Geometry: final body of the model. Coordinates: model frame, mm. Give positions to 0.01 mm unless a question says otherwise; leave off trailing zeros. Write each loop counter-clockwise with the first axis right and the second up, starting at its lowest first coordinate (ties: lowest second). Pieces come first, ordered by that corner, then holes. Notation, with made-up numbers: (14.5, 50.25) -> (60.5, 50.25) arc R27 ccw to (60.5, 69.25) -> close; hole circle Ø2 at (86, 23.5). An arc over 180 degrees is marked (long way). Answer as a JSON object with one key per item and string values. Group by question number.
(1) Contact query for flat-ended pins moving along their axis: pin 1 Ø3 at (x, z) = (40, -40) entering from -Y; pin 2 Ø6.5 at (x, z) = (-40, 40) entering from +Y; pin 3 Ø4.5 at (x, z) = (-100.5, -15.5) entering from -Y; pin 4 Ø1 at (x, y) = (188, 3.5) entering from +Z. Output: stop coordinate, or through.
(2) Draft query along X for faces 1 (the face through (61, 5, -1)), 2 (the face through (-104.846, 2.535, -1.465)), 3 (the face through (279, 2, -34)). Return one class per face: +X half, -X half, draft (parallel to the pull), parting line (faces both ways), or undercut.
(3) Section query A-A on y = 3.9. State how many separate pieces and enclosed holes the cut face has, plus the area to 3 significant figures.
(4) Section query B-B on x = 216. Output: boundary loops of the cut face in (y, z).
(5) Material intervals for probe 1 along Z at (x, y) = (-100.5, 2.5); probe 2 along X at (y, z) = (2.8, 15.5); probe 3 along X at (y, z) = (2.2, -1.5), sorted ascending.
(6) Section query C-C on x = 67. Output: boundary loops of the cut face in (y, z), plus the area to 3 significant figures.
from build123d import *

# Parameters (mm, degrees)
BOSS_EXTRUDE2_DEPTH                                 = 5
CHAMFER2_SIZE                                       = 12
FILLET1_R                                           = 7.5
SKETCH2_R                                           = 2.575
SKETCH2_R_2                                         = 11.25
SKETCH2_R_3                                         = 3
CUT_EXTRUDE1_DEPTH                                  = 290.39592257
CSK_FOR_M3_COUNTERSUNK_FLAT_HEAD_SCREW2_D           = 3.4
CSK_FOR_M3_COUNTERSUNK_FLAT_HEAD_SCREW2_CSINK_D     = 6.3
CSK_FOR_M3_COUNTERSUNK_FLAT_HEAD_SCREW2_CSINK_ANGLE = 90


with BuildPart() as part:
    # Sketch1 → Boss-Extrude2 (new body)
    with BuildSketch(Plane(origin=(0, 0, 0), x_dir=(1, 0, 0), z_dir=(0, 1, 0))):
        Polygon((40, -50), (77.320508076, -40), (285, -40), (285, 40), (77.320508076, 40), (40, 50), (-40, 50), (-157, 50), (-157, -50), (-40, -50), align=None)
    extrude(amount=BOSS_EXTRUDE2_DEPTH)

    # Chamfer2
    chamfer2_edges = [part.edges().sort_by_distance(p)[0] for p in [
        (-157, 2.5, 50),
        (-157, 2.5, -50),
        (285, 2.5, -40),
        (285, 2.5, 40),
    ]]
    chamfer(chamfer2_edges, length=CHAMFER2_SIZE)

    # Fillet1
    fillet1_edges = [part.edges().sort_by_distance(p)[0] for p in [
        (40, 2.5, -50),
        (77.320508076, 2.5, -40),
        (77.320508076, 2.5, 40),
        (40, 2.5, 50),
        (-145, 2.5, 50),
        (-157, 2.5, -38),
        (-157, 2.5, 38),
        (-145, 2.5, -50),
        (273, 2.5, -40),
        (285, 2.5, 28),
        (285, 2.5, -28),
        (273, 2.5, 40),
    ]]
    fillet(fillet1_edges, radius=FILLET1_R)

    # Sketch2 → Cut-Extrude1 (cut, through all)
    with BuildSketch(Plane(origin=(0, 5, 0), x_dir=(1, 0, 0), z_dir=(0, 1, 0))):
        with Locations(Location((-40, 40, 0), (0, 0, 270))):
            Circle(SKETCH2_R)
        with Locations(Location((40, 40, 0), (0, 0, 90))):
            Circle(SKETCH2_R)
        with Locations(Location((40, -40, 0), (0, 0, 270))):
            Circle(SKETCH2_R)
        with Locations(Location((-40, -40, 0), (0, 0, 90))):
            Circle(SKETCH2_R)
        with Locations(Location((-116, 0, 0), (0, 0, 270))):
            Circle(SKETCH2_R_2)
        with Locations(Location((0, 0, 0), (0, 0, 270))):
            Circle(SKETCH2_R_3)
    extrude(amount=-CUT_EXTRUDE1_DEPTH, mode=Mode.SUBTRACT)

    # CSK for M3 Countersunk Flat Head Screw2 (through all)
    with Locations(Plane(origin=(0, 0, 0), x_dir=(-1, 0, 0), z_dir=(0, -1, 0))):
        with Locations((131.5, 15.5), (131.5, -15.5), (100.5, -15.5), (100.5, 15.5)):
            CounterSinkHole(CSK_FOR_M3_COUNTERSUNK_FLAT_HEAD_SCREW2_D / 2, CSK_FOR_M3_COUNTERSUNK_FLAT_HEAD_SCREW2_CSINK_D / 2, counter_sink_angle=CSK_FOR_M3_COUNTERSUNK_FLAT_HEAD_SCREW2_CSINK_ANGLE)


solid = part.part
Answer list:
{
 "1": {"pin 1": "through", "pin 2": "y = 5", "pin 3": "y = 0.9", "pin 4": "z = 40"},
 "2": {"face 1": "draft", "face 2": "undercut", "face 3": "+X half"},
 "3": {"separate pieces": "1", "enclosed holes": "10", "area": "38,800 mm2"},
 "4": {"outline": "(0, -40) -> (5, -40) -> (5, 40) -> (0, 40) -> close"},
 "5": {"probe 1": "-50 to -17.2, -13.8 to 13.8, 17.2 to 50", "probe 2": "-157 to -133.2, -129.8 to -102.2, -98.8 to 285", "probe 3": "-157 to -127.15, -104.85 to -2.6, 2.6 to 285"},
 "6": {"outline": "(0, -42.77) -> (5, -42.77) -> (5, 42.77) -> (0, 42.77) -> close", "area": "428 mm2"}
}
